Verification items for the finished model (mm, model axes). A direction names the side the tool comes from. Round coordinates to 2 decimals unless told otherwise and drop trailing zeros. Write each loop counter-clockwise with the first axis right and the second up, starting at its lowest first coordinate (ties: lowest second). Pieces come first, ordered by that corner, then holes. Notation, with made-up numbers: (74.5, 15.25) - (130.5, 15.25) arc R32 cw to (130.5, 49.25) - close; hole circle Ø8 at (61.25, 6). An arc over 180 degrees is marked (long way). Answer as a JSON object with one key per item and string values.
```python
from build123d import *

# Parameters (mm, degrees)
BOSS_EXTRUDE1_DEPTH = 1.9
SKETCH2_W           = 6.499536779
SKETCH2_H           = 1.569153834
BOSS_EXTRUDE2_DEPTH = 0.1
BOSS_EXTRUDE3_START = -0.3
SKETCH3_W           = 0.2
SKETCH3_H           = 1
BOSS_EXTRUDE3_DEPTH = 0.5
SKETCH4_W           = 5.899073558
SKETCH4_H           = 2.069153834
CUT_EXTRUDE1_DEPTH  = 1.7
CHAMFER1_SIZE       = 0.1
SKETCH5_W           = 0.32618924
SKETCH5_H           = 0.2
CUT_EXTRUDE2_DEPTH  = 1.6
FILLET1_R           = 0.2
FILLET2_R           = 0.2
FILLET3_R           = 0.1


with BuildPart() as part:
    # Sketch1 → Boss-Extrude1 (new body)
    with BuildSketch(Plane.XY):
        with BuildLine():
            Line((3.25, -5.898632739), (-3.249536779, -5.898632739))
            Line((-3.249536779, -5.898632739), (-3.25, -10.655382732))
            ThreePointArc((-3.25, -10.655382732), (0, -8.117786573), (3.25, -10.655382732))
            Line((3.25, -10.655382732), (3.25, -5.898632739))
        make_face()
    extrude(amount=-BOSS_EXTRUDE1_DEPTH)

    # Sketch2 → Boss-Extrude2 (add)
    with BuildSketch(Plane(origin=(0, 0, -1.9), x_dir=(-1, 0, 0), z_dir=(0, 0, -1))):
        with Locations((-0.00023161, -6.683209656)):
            Rectangle(SKETCH2_W, SKETCH2_H)
    extrude(amount=BOSS_EXTRUDE2_DEPTH)

    # Sketch3 → Boss-Extrude3 (add)
    with BuildSketch(Plane.ZY.offset(3.249536779).offset(BOSS_EXTRUDE3_START)):
        with Locations((-2.1, -6.887362902)):
            Rectangle(SKETCH3_W, SKETCH3_H)
    boss_extrude3 = extrude(amount=BOSS_EXTRUDE3_DEPTH)

    # Mirror1: Boss-Extrude3 across plane
    add(boss_extrude3.mirror(Plane(origin=(0, 0, 0), x_dir=(0, 0, 1), z_dir=(1, 0, 0))))

    # Sketch4 → Cut-Extrude1 (cut)
    with BuildSketch(Plane(origin=(0, 0, -2), x_dir=(-1, 0, 0), z_dir=(0, 0, -1))):
        with Locations((0, -6.933209656)):
            Rectangle(SKETCH4_W, SKETCH4_H)
    extrude(amount=-CUT_EXTRUDE1_DEPTH, mode=Mode.SUBTRACT)

    # Chamfer1
    chamfer1_edges = [part.edges().sort_by_distance(p)[0] for p in [
        (-3.449536779, -6.887362902, -2.2),
        (3.449536779, -6.887362902, -2.2),
    ]]
    chamfer(chamfer1_edges, length=CHAMFER1_SIZE)

    # Sketch5 → Cut-Extrude2 (cut)
    with BuildSketch(Plane(origin=(0, 0, -1.9), x_dir=(-1, 0, 0), z_dir=(0, 0, -1))):
        with Locations((3.112631399, -7.567786573)):
            Rectangle(SKETCH5_W, SKETCH5_H)
        with Locations((-3.112631399, -7.567786573)):
            Rectangle(SKETCH5_W, SKETCH5_H)
    extrude(amount=-CUT_EXTRUDE2_DEPTH, mode=Mode.SUBTRACT)

    # Fillet1
    fillet1_edges = [part.edges().sort_by_distance(p)[0] for p in [
        (2.949536779, -6.683209656, -0.3),
        (2.949536779, -7.967786573, -1.1),
        (0, -7.967786573, -0.3),
        (-2.949536779, -7.967786573, -1.1),
        (-2.949536779, -7.817786573, -0.3),
        (-2.949536779, -6.683209656, -0.3),
        (2.949536779, -7.817786573, -0.3),
    ]]
    fillet(fillet1_edges, radius=FILLET1_R)

    # Fillet2
    fillet2_edges = [part.edges().sort_by_distance(p)[0] for p in [
        (-3.25, -10.655382732, -0.95),
        (3.25, -10.655382732, -0.95),
    ]]
    fillet(fillet2_edges, radius=FILLET2_R)

    # Fillet3
    # the kernel refuses this fillet: 0.1 mm, written as the material it takes off along each edge
    with BuildSketch(Plane(origin=(3.15, -5.998632739, -0.1), x_dir=(1, 0, 0), z_dir=(0, 0, 1))) as fillet3_piece_1_section:
        Polygon((0, 0), (FILLET3_R, 0), (FILLET3_R, FILLET3_R), (0, FILLET3_R), align=None)
    fillet3_piece_1 = extrude(amount=FILLET3_R, mode=Mode.PRIVATE)
    fillet3_piece_1 = fillet3_piece_1 - Plane(origin=(3.15, -5.998632739, -0.1), x_dir=(-0.7071067811865476, -0.7071067811865475, 0), z_dir=(0, 0, 1)) * Sphere(FILLET3_R, mode=Mode.PRIVATE)
    add(fillet3_piece_1, mode=Mode.SUBTRACT)
    with BuildSketch(Plane(origin=(-3.149546516, -5.998632739, -0.1), x_dir=(0, 1, 0), z_dir=(0, 0, 1))) as fillet3_piece_2_section:
        Polygon((0, 0), (FILLET3_R, 0), (FILLET3_R, FILLET3_R * 0.999902622813), (FILLET3_R * 9.738192815e-05, FILLET3_R * 0.999999995258), align=None)
    fillet3_piece_2 = extrude(amount=FILLET3_R, mode=Mode.PRIVATE)
    fillet3_piece_2 = fillet3_piece_2 - Plane(origin=(-3.149546516, -5.998632739, -0.1), x_dir=(0.7070723506374189, -0.7071412100592604, 0), z_dir=(0, 0, 1)) * Sphere(FILLET3_R, mode=Mode.PRIVATE)
    add(fillet3_piece_2, mode=Mode.SUBTRACT)
    with BuildSketch(Plane(origin=(3.25, -9.65119636, 0), x_dir=(-1, 0, 0), z_dir=(0, 1, 0))) as fillet3_piece_3:
        with BuildLine():
            CenterArc((FILLET3_R, -FILLET3_R), FILLET3_R, 90, 90)
            Line((0, -FILLET3_R), (0, 0))
            Line((0, 0), (FILLET3_R, 0))
        make_face()
    extrude(amount=3.652563621, mode=Mode.SUBTRACT)
    with BuildSketch(Plane(origin=(3.05, -9.65119636, 0), x_dir=(-0.8591549295774534, -0.511715552805229, 0), z_dir=(-0.511715552805229, 0.8591549295774534, 0))) as fillet3_piece_4:
        with BuildLine():
            CenterArc((0.2 - FILLET3_R, -FILLET3_R), FILLET3_R, 0, 90)
            Line((0.2, -FILLET3_R), (0.2, 0))
            Line((0.2, 0), (0.2 - FILLET3_R, 0))
        make_face()
    revolve(axis=Axis((3.05, -9.65119636, 0), (0, 0, 1)), revolution_arc=149.221830438, mode=Mode.SUBTRACT)
    with BuildSketch(Plane(origin=(0, -11.467786573, 0), x_dir=(-0.8591273784381983, 0.5117618075021901, 0), z_dir=(-0.5117618075021901, -0.8591273784381983, 0))) as fillet3_piece_5:
        with BuildLine():
            CenterArc((3.35 + FILLET3_R, FILLET3_R), FILLET3_R, 180, 90)
            Line((3.35, FILLET3_R), (3.35, 0))
            Line((3.35, 0), (3.35 + FILLET3_R, 0))
        make_face()
    revolve(axis=Axis((0, -11.467786573, 0), (0, 0, -1)), revolution_arc=118.440576169, mode=Mode.SUBTRACT)
    with BuildSketch(Plane(origin=(-3.049902193, -9.651032156, 0), x_dir=(0.8591273784382029, -0.5117618075021826, 0), z_dir=(0.5117618075021826, 0.8591273784382029, 0))) as fillet3_piece_6:
        with BuildLine():
            CenterArc((0.2 - FILLET3_R, FILLET3_R), FILLET3_R, 270, 90)
            Line((0.2, FILLET3_R), (0.2, 0))
            Line((0.2, 0), (0.2 - FILLET3_R, 0))
        make_face()
    revolve(axis=Axis((-3.049902193, -9.651032156, 0), (0, 0, -1)), revolution_arc=149.224325304, mode=Mode.SUBTRACT)
    with BuildSketch(Plane(origin=(-3.249546516, -5.998623001, 0), x_dir=(0.99999999525838, -9.738192814999169e-05, 0), z_dir=(-9.73819281499917e-05, -0.9999999952583801, 0))) as fillet3_piece_7:
        with BuildLine():
            CenterArc((FILLET3_R, -FILLET3_R), FILLET3_R, 90, 90)
            Line((0, -FILLET3_R), (0, 0))
            Line((0, 0), (FILLET3_R, 0))
        make_face()
    extrude(amount=3.652389696, mode=Mode.SUBTRACT)
    with BuildSketch(Plane(origin=(3.25, -5.898632739, -0.1), x_dir=(0, -1, 0), z_dir=(0, 0, -1))) as fillet3_piece_8:
        with BuildLine():
            CenterArc((FILLET3_R, FILLET3_R), FILLET3_R, 180, 90)
            Line((0, FILLET3_R), (0, 0))
            Line((0, 0), (FILLET3_R, 0))
        make_face()
    extrude(amount=1.8, mode=Mode.SUBTRACT)
    with BuildSketch(Plane(origin=(3.15, -5.898632739, 0), x_dir=(0, -1, 0), z_dir=(-1, 0, 0))) as fillet3_piece_9:
        with BuildLine():
            CenterArc((FILLET3_R, -FILLET3_R), FILLET3_R, 90, 90)
            Line((0, -FILLET3_R), (0, 0))
            Line((0, 0), (FILLET3_R, 0))
        make_face()
    extrude(amount=6.299546516, mode=Mode.SUBTRACT)
    with BuildSketch(Plane(origin=(-3.249536779, -5.898632739, -0.1), x_dir=(1, 0, 0), z_dir=(0, 0, -1))) as fillet3_piece_10:
        with BuildLine():
            CenterArc((FILLET3_R * 0.999902622813, FILLET3_R), FILLET3_R, 180.005579573, 89.994420427)
            Line((-FILLET3_R * 9.73724453734e-05, FILLET3_R * 0.999902618072), (0, 0))
            Line((0, 0), (FILLET3_R * 0.999902622813, 0))
        make_face()
    extrude(amount=1.8, mode=Mode.SUBTRACT)
    with BuildSketch(Plane(origin=(-3.249536779, -5.898632739, -1.9), x_dir=(1.0, -4.7416204296268874e-09, 0), z_dir=(0, 0, -1)), Plane(origin=(3.25, -5.898632739, -1.9), x_dir=(0, -1, 0), z_dir=(0, 0, -1))) as fillet3_piece_11:
        with BuildLine():
            CenterArc((FILLET3_R * 1.00000000474, FILLET3_R), FILLET3_R, 179.999999728, 90)
            Line((FILLET3_R * 4.74162045211e-09, FILLET3_R * 1.00000000474), (0, 0))
            Line((0, 0), (FILLET3_R, 0))
        make_face()
    extrude(amount=0.350000001, mode=Mode.SUBTRACT)
    with BuildSketch(Plane(origin=(-3.49953678, -5.898632739, -2), x_dir=(0, -4.7416204296268874e-09, 1.0), z_dir=(1, 0, 0))) as fillet3_piece_12:
        with BuildLine():
            CenterArc((FILLET3_R * 1.00000000474, FILLET3_R), FILLET3_R, 179.999999728, 90)
            Line((FILLET3_R * 4.74162045211e-09, FILLET3_R * 1.00000000474), (0, 0))
            Line((0, 0), (FILLET3_R, 0))
        make_face()
    extrude(amount=0.800000002, mode=Mode.SUBTRACT)
    with BuildSketch(Plane(origin=(-2.949536779, -5.898632739, -2.250000001), x_dir=(-1.0, -4.7416204296268874e-09, 0), z_dir=(0, 0, 1))) as fillet3_piece_13:
        with BuildLine():
            CenterArc((FILLET3_R * 1.00000000474, FILLET3_R), FILLET3_R, 179.999999728, 90)
            Line((FILLET3_R * 4.74162045211e-09, FILLET3_R * 1.00000000474), (0, 0))
            Line((0, 0), (FILLET3_R, 0))
        make_face()
    extrude(amount=1.750000001, mode=Mode.SUBTRACT)
    with BuildSketch(Plane(origin=(-2.749536779, -5.898632739, -0.5), x_dir=(0, 0, 1), z_dir=(1, 0, 0))) as fillet3_piece_14:
        with BuildLine():
            CenterArc((0.2 + FILLET3_R, FILLET3_R), FILLET3_R, 180, 90)
            Line((0.2, FILLET3_R), (0.2, 0))
            Line((0.2, 0), (0.2 + FILLET3_R, 0))
        make_face()
    revolve(axis=Axis((-2.749536779, -5.898632739, -0.5), (0, -1, 0)), revolution_arc=90, mode=Mode.SUBTRACT)
    with BuildSketch(Plane(origin=(-2.749536779, -5.898632739, -0.3), x_dir=(0, -4.7416204296268916e-09, 1.0), z_dir=(1, 0, 0))) as fillet3_piece_15:
        with BuildLine():
            CenterArc((FILLET3_R * 1.00000000474, FILLET3_R), FILLET3_R, 179.999999728, 90)
            Line((FILLET3_R * 4.74162045211e-09, FILLET3_R * 1.00000000474), (0, 0))
            Line((0, 0), (FILLET3_R, 0))
        make_face()
    extrude(amount=5.499073557, mode=Mode.SUBTRACT)
    with BuildSketch(Plane(origin=(2.749536779, -5.898632739, -0.5), x_dir=(0, 0, 1), z_dir=(-1, 0, 0))) as fillet3_piece_16:
        with BuildLine():
            CenterArc((0.2 + FILLET3_R, -FILLET3_R), FILLET3_R, 90, 90)
            Line((0.2, -FILLET3_R), (0.2, 0))
            Line((0.2, 0), (0.2 + FILLET3_R, 0))
        make_face()
    revolve(axis=Axis((2.749536779, -5.898632739, -0.5), (0, 1, 0)), revolution_arc=90, mode=Mode.SUBTRACT)
    with BuildSketch(Plane(origin=(2.949536779, -5.898632739, -2.250000001), x_dir=(1.0, -4.7416204296268874e-09, 0), z_dir=(0, 0, 1))) as fillet3_piece_17:
        with BuildLine():
            CenterArc((FILLET3_R * 1.00000000474, -FILLET3_R), FILLET3_R, 90.000000272, 90)
            Line((FILLET3_R * 4.74162045211e-09, -FILLET3_R * 1.00000000474), (0, 0))
            Line((0, 0), (FILLET3_R, 0))
        make_face()
    extrude(amount=1.750000001, mode=Mode.SUBTRACT)
    with BuildSketch(Plane(origin=(2.699536777, -5.898632739, -2), x_dir=(0, -4.7416204296268874e-09, 1.0), z_dir=(1, 0, 0))) as fillet3_piece_18:
        with BuildLine():
            CenterArc((FILLET3_R * 1.00000000474, FILLET3_R), FILLET3_R, 179.999999728, 90)
            Line((FILLET3_R * 4.74162045211e-09, FILLET3_R * 1.00000000474), (0, 0))
            Line((0, 0), (FILLET3_R, 0))
        make_face()
    extrude(amount=0.800463224, mode=Mode.SUBTRACT)


solid = part.part
```
1. Material ranges on probe 1 along X at (y, z) = (-7.4, -1.1); probe 2 along Z at (x, y) = (-1.5, -6.5); probe 3 along X at (y, z) = (-8.95, -0.85), recorded low to high. Write a range as from..to.
Completed:
{"probe 1": "x = -3.25..-2.95, 2.95..3.25", "probe 2": "z = -0.3..0", "probe 3": "x = -3.25..-2.21, 2.21..3.25"}
2. Go/stop test with flat-tipped pins: pin 1 (0.9 mm diameter, centred on x = -1, y = -6.5, fed in from -Z); pin 2 (1 mm diameter, centred on y = -9, z = -0.5, fed in from +X); pin 3 (0.5 mm diameter, centred on y = -7, z = -0.5, fed in from -X). Record where each tip stops, or that it passes through.
Completed:
{"pin 1": "stops at z = -0.3", "pin 2": "stops at x = 3.25", "pin 3": "stops at x = -3.25"}
3. Access from +Z, -Z, +X, -X, +Y, -Y to the whole of each face (thin tool, end or side, straight path). Record for faces 1 (the face through (2.95, -7, -1)), 2 (the face through (-0.05, -8.12, -0.99)).
Completed:
{"face 1": "-Z, +Y", "face 2": "+Z, -Z, -Y"}
4. Cross-section at A-A (z = -1.8). Record the boundary of the cut face in (x, y), plus the area to 3 significant figures.
Completed:
{"outline": "(-3.25, -9.65) arc R0.2 ccw to (-2.88, -9.75) arc R3.35 cw to (2.88, -9.75) arc R0.2 ccw to (3.25, -9.65) - (3.25, -7.67) - (2.95, -7.67) - (2.95, -7.77) arc R0.2 cw to (2.75, -7.97) - (-2.75, -7.97) arc R0.2 cw to (-2.95, -7.77) - (-2.95, -7.67) - (-3.25, -7.67) - close; (-3.25, -7.47) - (-2.95, -7.47) - (-2.95, -6) arc R0.1 ccw to (-3.05, -5.9) - (-3.15, -5.9) arc R0.1 ccw to (-3.25, -6) - close; (2.95, -7.47) - (3.25, -7.47) - (3.25, -6) arc R0.1 ccw to (3.15, -5.9) - (3.05, -5.9) arc R0.1 ccw to (2.95, -6) - close", "area": "6.12 mm^2"}
5. Mould release check, pull along X, two halves, no side actions. Record for faces 3 (the face through (-1.5, -8.3, -1.9)), 4 (the face through (3.25, -8, -1)), 5 (the face through (-2.95, -7, -1)), 6 (the face through (0, -7, -0.3)): released by +X, released by -X, zero draft, split by the parting line, or undercut.
Completed:
{"face 3": "zero draft", "face 4": "released by +X", "face 5": "undercut", "face 6": "undercut"}
